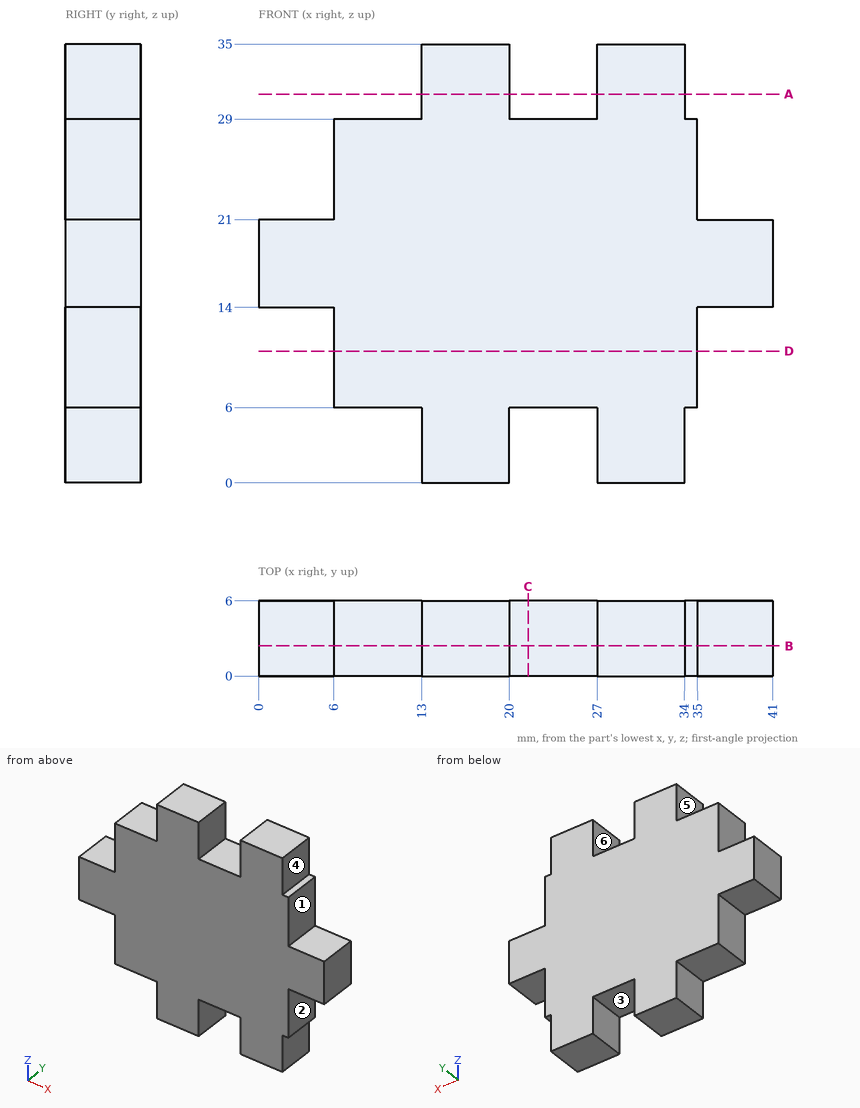
Study the drawing (mm; zero at the part's minimum x, y, z) and answer. A direction names the side the tool comes from. Give positions to 0.01 mm unless a question says otherwise; leave off trailing zeros. Order: outer loops, then holes, each group sorted by start corner. A loop starts at its lowest first (then second) coordinate and runs counter-clockwise, first axis right, second up. Notation, with made-up numbers: (47.5, 44.25) - (102.5, 44.25) arc R22 cw to (102.5, 54.25) - close; hole circle Ø3 at (-4.5, 51). An arc over 180 degrees is marked (long way). Use one line per item in the form item = value. Start each with the question number.
(1) For the marked faces 1, 2 and 3, determine the directions among +Z, -Z, +X, -X, +Y, -Y from which every point of the face is accessible in a straight line to the end or side of a thin tool.
(2) A cutting plane is placed at B-B, the plane y = 2.4. Write down the section's boundary in (x, z).
(3) Flat-ended cylindrical pins translate along their axes: pin 1 Ø3 at (y, z) = (4, 8) entering from +X; pin 2 Ø3 at (y, z) = (2, 3) entering from -X; pin 3 Ø1.5 at (x, y) = (23.5, 1.5) entering from -Z. Find the tip coordinate at first contact, or state that the pin passes through.
(4) A cutting plane is placed at D-D, the plane z = 10.5. Write down the section's boundary in (x, y).
(5) Consider line 1 (X direction, y = 2, z = 28.5); line 2 (X direction, y = 1.5, z = 30); line 3 (Z direction, x = 22, y = 2.2). Determine where each line is inside the solid, lowest interval first. Write a range as from..to.
(6) A cutting plane is placed at C-C, the plane x = 21.5. Write down the section's boundary in (y, z), then the cut area to 3 significant figures.
(7) A cutting plane is placed at A-A, the plane z = 31. Write down the section's boundary in (x, y), then the cut area to 3 significant figures.
(8) The mould has two halves that part along X. Classify the marked faces 4, 5 and 6: released by +X, released by -X, zero draft, split by the parting line, or undercut.
Ans:
q1.face_1 = +Z, +X, +Y, -Y
q1.face_2 = -Z, +X, +Y, -Y
q1.face_3 = -Z, +Y, -Y
q2.outline = (0, 14) - (6, 14) - (6, 6) - (13, 6) - (13, 0) - (20, 0) - (20, 6) - (27, 6) - (27, 0) - (34, 0) - (34, 6) - (35, 6) - (35, 14) - (41, 14) - (41, 21) - (35, 21) - (35, 29) - (34, 29) - (34, 35) - (27, 35) - (27, 29) - (20, 29) - (20, 35) - (13, 35) - (13, 29) - (6, 29) - (6, 21) - (0, 21) - close
q3.pin_1 = 35
q3.pin_2 = 13
q3.pin_3 = 6
q4.outline = (6, 0) - (35, 0) - (35, 6) - (6, 6) - close
q5.line_1 = 6..35
q5.line_2 = 13..20, 27..34
q5.line_3 = 6..29
q6.outline = (0, 6) - (6, 6) - (6, 29) - (0, 29) - close
q6.area = 138 mm^2
q7.outline = (13, 0) - (20, 0) - (20, 6) - (13, 6) - close; (27, 0) - (34, 0) - (34, 6) - (27, 6) - close
q7.area = 84.0 mm^2
q8.face_4 = released by +X
q8.face_5 = released by -X
q8.face_6 = undercut
